```python
from build123d import *

# Parameters (mm, degrees)
F0_W     = 1016
F0_H     = 101.6
F0_R     = 30.1244
F1_DEPTH = 19.05
F2_W     = 19.05
F2_H     = 50.8
F3_DEPTH = 13.97


with BuildPart() as f1:
    # F0 (on Top) → F1 (new body)
    with BuildSketch(Plane.XY):
        with Locations((-508, -50.8)):
            Rectangle(F0_W, F0_H)
        with Locations((-935.0756, -50.8)):
            Circle(F0_R, mode=Mode.SUBTRACT)
    extrude(amount=F1_DEPTH)

    # F2 (on face) → F3 (cut)
    with BuildSketch(Plane.XY.offset(19.05)):
        with Locations((-60.325, -50.8)):
            Rectangle(F2_W, F2_H)
    extrude(amount=-F3_DEPTH, mode=Mode.SUBTRACT)


solid = f1.part
```
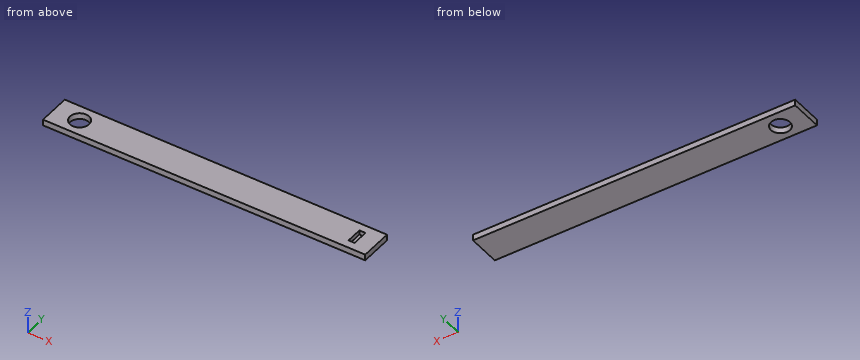
Read the model definition and answer for the solid it produces. Units are mm, in the model's axes. Coordinates: 2 decimals unless noted, no trailing zeros. Loops run counter-clockwise (first coordinate to the right, second up) from the corner with the lowest first, then second, coordinate; pieces in that order, holes last. Notation, with made-up numbers: (37.25, -14.75) -> (58.25, -14.75) arc R23 ccw to (58.25, 7.25) -> close; hole circle Ø7 at (10.5, 67.25). An arc over 180 degrees is marked (long way). Return JSON: item names as keys, results as strings.
Item 1: Find section A-A (y = -50.8). Determine the outline of the cut face in (x, z), plus the area to 3 significant figures.
Answers:
{"outline": "(-1016, 0) -> (-965.2, 0) -> (-965.2, 19.05) -> (-1016, 19.05) -> close; (-904.95, 0) -> (0, 0) -> (0, 19.05) -> (-50.8, 19.05) -> (-50.8, 5.08) -> (-69.85, 5.08) -> (-69.85, 19.05) -> (-904.95, 19.05) -> close", "area": "17,900 mm2"}
Item 2: Find section B-B (z = 13.5). Determine the outline of the cut face in (x, y), plus the area to 3 significant figures.
Answers:
{"outline": "(-1016, -101.6) -> (0, -101.6) -> (0, 0) -> (-1016, 0) -> close; hole circle Ø60.25 at (-935.08, -50.8); hole (-69.85, -76.2) -> (-50.8, -76.2) -> (-50.8, -25.4) -> (-69.85, -25.4) -> close", "area": "99,400 mm2"}
Item 3: Find section C-C (x = -924). Determine the outline of the cut face in (y, z), plus the area to 3 significant figures.
Answers:
{"outline": "(-101.6, 0) -> (-78.81, 0) -> (-78.81, 19.05) -> (-101.6, 19.05) -> close; (-22.79, 0) -> (0, 0) -> (0, 19.05) -> (-22.79, 19.05) -> close", "area": "868 mm2"}
Item 4: Find the intervals of material crossed by probe 1 along X at (y, z) = (-48, 7.75); probe 2 along X at (y, z) = (-63, 18.25); probe 3 along Y at (x, z) = (-69, 11.5), in increasing order.
Answers:
{"probe 1": "x = -1016 to -965.07, -905.08 to -69.85, -50.8 to 0", "probe 2": "x = -1016 to -962.62, -907.53 to -69.85, -50.8 to 0", "probe 3": "y = -101.6 to -76.2, -25.4 to 0"}
Item 5: A flat-ended cylindrical pin translates along its axis: P1, Ø9.5, axis at x = -59.5, y = -63, coming from the +Z side. Find the tip coordinate at first contact, or state that the pin passes through.
Answers:
{"P1": "stops at z = 5.08"}
